Input: part model. Units: mm. Frame: model coordinates. Round coordinates to 2 decimals unless told otherwise and drop trailing zeros. Order: outer loops, then holes, each group sorted by start corner. A loop starts at its lowest first (then second) coordinate and runs counter-clockwise, first axis right, second up.
Item 1: Cut plane A-A on z = 70. Output: boundary loops of the cut face in (x, y).
Item 2: First-contact query: pin 1 (1 mm diameter, centred on x = 140.5, y = -1, fed in from -Z); pin 2 (1 mm diameter, centred on y = -0.5, z = 75.5, fed in from -X). Flat tips, straight axial feed; report the tip coordinate or a pass-through.
Item 3: Line query: L1, parallel to X at y = -1.75, z = 37.5; L2, parallel to X at y = -0.25, z = 91; L3, parallel to Z at x = 204, y = -0.8. Output: solid intervals per line, ascending.
Item 4: Cut plane B-B on y = -1.4. Give the number of separate pieces and of enclosed holes in the cut face, then the cut area to 3 significant figures.
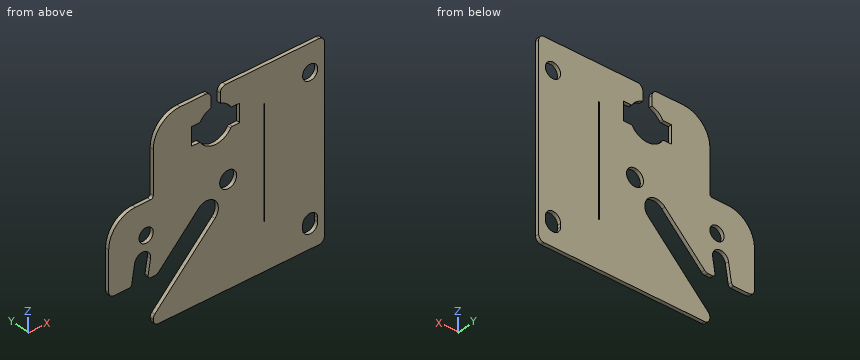
```python
from build123d import *

# Parameters (mm, degrees)
F0_R     = 4
F0_R_2   = 4.75
F0_W     = 0.5
F0_H     = 60
F0_R_3   = 4.25
F1_DEPTH = 2
F2_R     = 15
F3_R     = 3
F4_R     = 1.5
F5_R     = 1


# Not quite as in the source:
# - a feature names something its author has since deleted; it is built from what else it names


with BuildPart() as f1:
    # F0 (on Front) → F1 (new body)
    with BuildSketch(Plane.XZ):
        with BuildLine():
            Line((159.6967741251, 4.7991039181), (159.6967741251, 0))
            Line((159.6967741251, 0), (255.6967741251, 0))
            Line((255.6967741251, 0), (255.6967741251, 105))
            Line((255.6967741251, 105), (197.2967741251, 105))
            Line((197.2967741251, 105), (197.2967741251, 96.7078576421))
            ThreePointArc((197.2967741251, 96.7078576421), (200.8257976645, 94.9647705839), (203.4147153958, 92))
            Line((203.4147153958, 92), (208.1967741251, 92))
            Line((208.1967741251, 92), (208.1967741251, 82))
            Line((208.1967741251, 82), (203.4147153958, 82))
            ThreePointArc((203.4147153958, 82), (194.6967741251, 76.95), (185.9788328544, 82))
            Line((185.9788328544, 82), (181.1967741251, 82))
            Line((181.1967741251, 82), (181.1967741251, 92))
            Line((181.1967741251, 92), (185.9788328544, 92))
            ThreePointArc((185.9788328544, 92), (188.5677505857, 94.9647705839), (192.0967741251, 96.7078576421))
            Line((192.0967741251, 96.7078576421), (192.0967741251, 105))
            Line((192.0967741251, 105), (159.6967741251, 105))
            Line((159.6967741251, 105), (159.6967741251, 65))
            Line((159.6967741251, 65), (134.6967741251, 65))
            Line((134.6967741251, 65), (134.6967741251, 25.3155251003))
            Line((134.6967741251, 25.3155251003), (147.4130505224, 25.3155251003))
            Line((147.4130505224, 25.3155251003), (149.2561978018, 36.5444159815))
            ThreePointArc((149.2561978018, 36.5444159815), (154.4256650063, 40.2561014236), (158.1373504484, 35.0866342191))
            Line((158.1373504484, 35.0866342191), (156.5334882879, 25.3155251003))
            Line((156.5334882879, 25.3155251003), (161.81991107, 25.3155251003))
            Line((161.81991107, 25.3155251003), (163.0631786775, 26.5587927078))
            Line((163.0631786775, 26.5587927078), (184.9027867776, 48.3984008079))
            ThreePointArc((184.9027867776, 48.3984008079), (194.1972390474, 48.6983039321), (194.2972221661, 39.399551959))
            Line((194.2972221661, 39.399551959), (159.6967741251, 4.7991039181))
        make_face()
        with Locations((155.6967741251, 48)):
            Circle(F0_R, mode=Mode.SUBTRACT)
        with BuildLine():
            ThreePointArc((251.9467741251, 12), (247.6967741251, 7.75), (243.4467741251, 12))
            Line((243.4467741251, 12), (243.4467741251, 14))
            ThreePointArc((243.4467741251, 14), (247.6967741251, 18.25), (251.9467741251, 14))
            Line((251.9467741251, 14), (251.9467741251, 12))
        make_face(mode=Mode.SUBTRACT)
        with Locations((201.6967741251, 56)):
            Circle(F0_R_2, mode=Mode.SUBTRACT)
        with Locations((221.9467741251, 55.5368482322)):
            Rectangle(F0_W, F0_H, mode=Mode.SUBTRACT)
        with Locations((247.6967741251, 90)):
            Circle(F0_R_3, mode=Mode.SUBTRACT)
    extrude(amount=F1_DEPTH)

    # F2
    f2_edges = [f1.edges().sort_by_distance(p)[0] for p in [
        (134.696774, -1, 65),
        (159.696774, -1, 105),
    ]]
    fillet(f2_edges, radius=F2_R)

    # F3
    f3_edges = [f1.edges().sort_by_distance(p)[0] for p in [
        (255.696774, -1, 105),
        (255.696774, -1, 0),
        (197.296774, -1, 105),
        (192.096774, -1, 105),
        (161.819911, -1, 25.315525),
        (159.696774, -1, 4.799104),
        (159.696774, -1, 0),
        (134.696774, -1, 25.315525),
    ]]
    fillet(f3_edges, radius=F3_R)

    # F4
    f4_edges = [f1.edges().sort_by_distance(p)[0] for p in [
        (147.413051, -1, 25.315525),
        (156.533488, -1, 25.315525),
        (159.696774, -1, 65),
    ]]
    fillet(f4_edges, radius=F4_R)

    # F5
    f5_edges = [f1.edges().sort_by_distance(p)[0] for p in [
        (185.978833, -1, 92),
        (185.978833, -1, 82),
        (203.414715, -1, 92),
        (203.414715, -1, 82),
    ]]
    fillet(f5_edges, radius=F5_R)


solid = f1.part
```
From the geometry:
1. outline: (159.7, -2) - (221.7, -2) - (221.7, 0) - (159.7, 0) - close; (222.2, -2) - (255.7, -2) - (255.7, 0) - (222.2, 0) - close
2. pin 1: stops at z = 25.32
2. pin 2: stops at x = 159.7
3. L1: x = 134.7 to 149.52, 157.87 to 174, 192.4 to 221.7, 222.2 to 255.7
3. L2: x = 159.73 to 181.2, 208.2 to 243.57, 251.83 to 255.7
3. L3: z = 0 to 51.85, 60.15 to 82, 92 to 105
4. separate pieces: 1
4. enclosed holes: 5
4. area: 9,500 mm2
